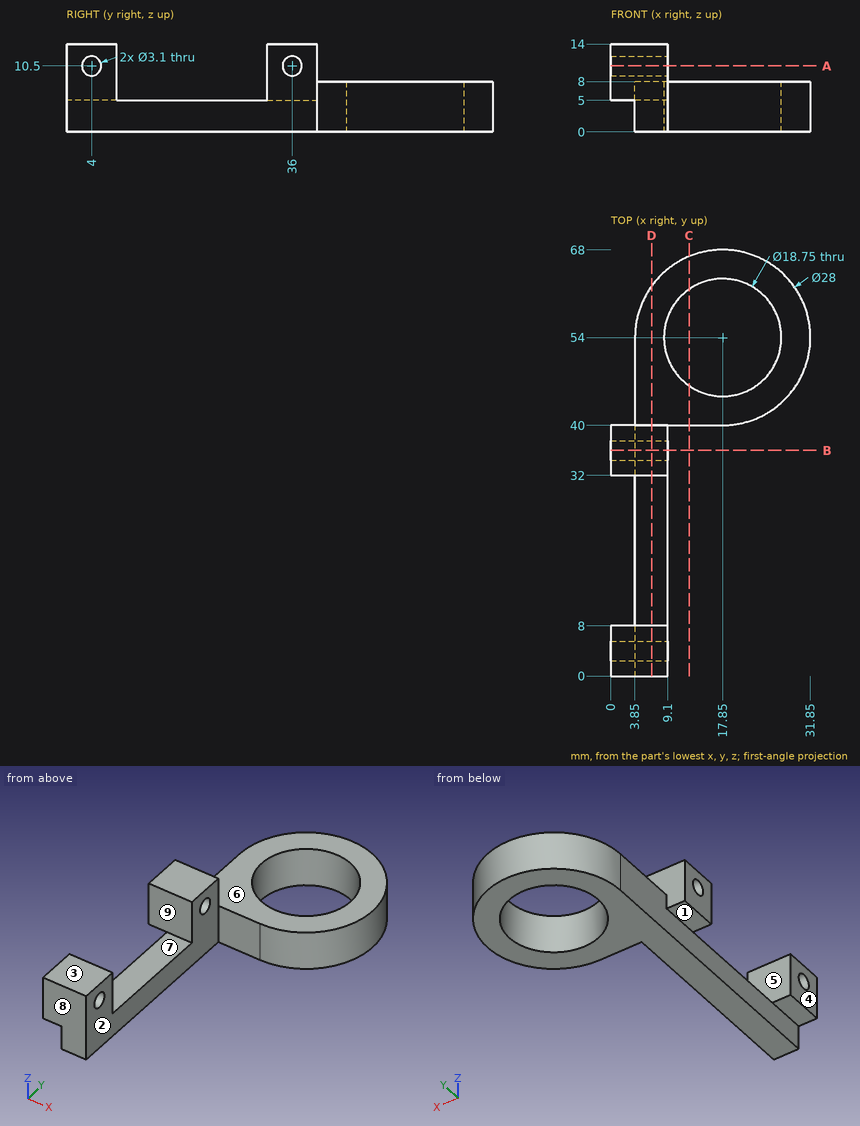
Input: dimensioned drawing with shaded views. Units: mm. Origin: part minimum x, y, z. A direction names the side the tool comes from. Give positions to 0.01 mm unless a question says otherwise; leave off trailing zeros. Loops run counter-clockwise (first coordinate to the right, second up) from the corner with the lowest first, then second, coordinate; pieces in that order, holes last. Notation, with made-up numbers: (57.25, 39.5) -> (75.25, 39.5) arc R26 cw to (75.25, 67.5) -> close; hole circle Ø6 at (-2, 70.25). An arc over 180 degrees is marked (long way). Use a Markdown table: item, result. Add a question column.
1) Section query C-C, the plane x = 12.5. Return the cut outline in (y, z), then the cut area to 3 significant figures.
2) Section query D-D, the plane x = 6.5. Return the cut outline in (y, z), then the cut area to 3 significant figures.
3) Reachability of the marked faces 1, 2, 3, 4 and 5 from +Z, -Z, +X, -X, +Y, -Y: full face, straight path, thin tool, end or side. Return the list, or none.
4) First-contact query: pin 1 (1.5 mm diameter, centred on y = 48.5, z = 8.5, fed in from -X); pin 2 (1.5 mm diameter, centred on x = 9, z = 11, fed in from +Y); pin 3 (6 mm diameter, centred on x = 7.5, y = 20, fed in from +Z). Flat tips, straight axial feed; report the tip coordinate or a pass-through.
5) Section query B-B, the plane y = 36. Return the cut outline in (x, z).
6) Pull-direction query (Y, two-part tool) for the marked faces 6, 7, 8 and 9; classes: +Y half, -Y half, draft (parallel to the pull), parting line (faces both ways), or undercut.
7) Line query: line 1 along Y through (x, z) = (17.85, 5.5) (3 decimals); line 2 along Z through (x, y) = (2.5, 36); line 3 along Z through (x, y) = (6.5, 36). Output: solid intervals per line, ascending. Write a range as [from, to].
8) Section query A-A, the plane z = 10.5. Return the cut outline in (x, y).
Numbers:
| question | item | result |
|---|---|---|
| 1 | outline | (40, 0) -> (46.3, 0) -> (46.3, 8) -> (40, 8) -> close; (61.7, 0) -> (66.94, 0) -> (66.94, 8) -> (61.7, 8) -> close |
| 1 | area | 92.3 mm2 |
| 2 | outline | (0, 0) -> (62.2, 0) -> (62.2, 8) -> (40, 8) -> (40, 14) -> (32, 14) -> (32, 5) -> (8, 5) -> (8, 14) -> (0, 14) -> close; hole circle Ø3.1 at (4, 10.5); hole circle Ø3.1 at (36, 10.5) |
| 2 | area | 506 mm2 |
| 3 | face 1 | -Z, -X, +Y, -Y |
| 3 | face 2 | +Z, -Z, +X, -Y |
| 3 | face 3 | +Z, +X, -X, +Y, -Y |
| 3 | face 4 | +Z, -Z, -X, +Y, -Y |
| 3 | face 5 | +Z, +X, -X |
| 4 | pin 1 | stops at x = 3.85 |
| 4 | pin 2 | stops at y = 40 |
| 4 | pin 3 | stops at z = 5 |
| 5 | outline | (0, 5) -> (3.85, 5) -> (3.85, 0) -> (9.1, 0) -> (9.1, 8.95) -> (0, 8.95) -> close; (0, 12.05) -> (9.1, 12.05) -> (9.1, 14) -> (0, 14) -> close |
| 6 | face 6 | draft |
| 6 | face 7 | undercut |
| 6 | face 8 | -Y half |
| 6 | face 9 | undercut |
| 7 | line 1 | y = [40, 44.625], [63.375, 68] |
| 7 | line 2 | z = [5, 8.95], [12.05, 14] |
| 7 | line 3 | z = [0, 8.95], [12.05, 14] |
| 8 | outline | (0, 0) -> (9.1, 0) -> (9.1, 2.45) -> (0, 2.45) -> close; (0, 5.55) -> (9.1, 5.55) -> (9.1, 8) -> (0, 8) -> close; (0, 32) -> (9.1, 32) -> (9.1, 34.45) -> (0, 34.45) -> close; (0, 37.55) -> (9.1, 37.55) -> (9.1, 40) -> (0, 40) -> close |
